The model under review builds one solid part; all positions refer to its coordinate system, in mm. Face numbers are marked on the shaded views. Coordinates: 2 decimals unless noted, no trailing zeros. Write each loop counter-clockwise with the first axis right and the second up, starting at its lowest first coordinate (ties: lowest second). Pieces come first, ordered by that corner, then holes. Notation, with made-up numbers: M 5.25,30 L 50.25,30 A10 ccw 50.25,46 Z; hole C 15.25,15.5 d6. An arc over 180 degrees is marked long. Answer as a JSON object with one key per item and string values.
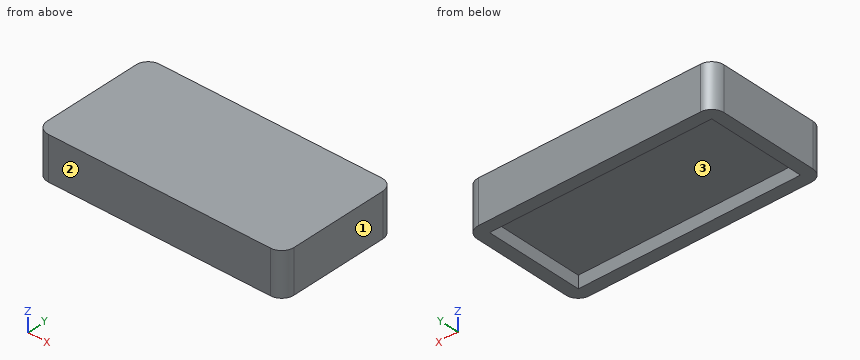
```python
from build123d import *

# Parameters (mm, degrees)
BOSS_EXTRUDE1_DEPTH = 3.5
SKETCH2_W           = 18
SKETCH2_H           = 8
CUT_EXTRUDE1_DEPTH  = 1


with BuildPart() as part:
    # Sketch1 → Boss-Extrude1 (new body)
    with BuildSketch(Plane.XY):
        with BuildLine():
            Line((-9, 5), (9, 5))
            ThreePointArc((9, 5), (9.707106781, 4.707106781), (10, 4))
            Line((10, 4), (10, -4))
            ThreePointArc((10, -4), (9.707106781, -4.707106781), (9, -5))
            Line((9, -5), (-9, -5))
            ThreePointArc((-9, -5), (-9.707106781, -4.707106781), (-10, -4))
            Line((-10, -4), (-10, 4))
            ThreePointArc((-10, 4), (-9.707106781, 4.707106781), (-9, 5))
        make_face()
    extrude(amount=BOSS_EXTRUDE1_DEPTH)

    # Sketch2 → Cut-Extrude1 (cut)
    with BuildSketch(Plane(origin=(0, 0, 0), x_dir=(-1, 0, 0), z_dir=(0, 0, -1))):
        Rectangle(SKETCH2_W, SKETCH2_H)
    extrude(amount=-CUT_EXTRUDE1_DEPTH, mode=Mode.SUBTRACT)


solid = part.part
```
(1) Add section C-C on y = 0.5. Give the boundary of the cut face in (x, z).
Results list:
{"outline": "M -10,0 L -9,0 L -9,1 L 9,1 L 9,0 L 10,0 L 10,3.5 L -10,3.5 Z"}
(2) Add section B-B on z = 0.4. Give the boundary of the cut face in (x, y), and give its area (3 significant figures).
Results list:
{"outline": "M -10,-4 A1 ccw -9,-5 L 9,-5 A1 ccw 10,-4 L 10,4 A1 ccw 9,5 L -9,5 A1 ccw -10,4 Z; hole M -9,-4 L 9,-4 L 9,4 L -9,4 Z", "area": "55.1 mm²"}
(3) Draft analysis for pull direction X (two halves, no side actions). For the marked faces 1, 2 and 3, state which applies: released by +X, released by -X, zero draft, split by the parting line, or undercut.
Results list:
{"face 1": "released by +X", "face 2": "zero draft", "face 3": "undercut"}
(4) Add section A-A on x = -4. Give the boundary of the cut face in (y, z).
Results list:
{"outline": "M -5,0 L -4,0 L -4,1 L 4,1 L 4,0 L 5,0 L 5,3.5 L -5,3.5 Z"}
(5) Wall thickness on line 1 along X through (y, z) = (-0.5, 0.5); line 2 along Y through (x, z) = (-7.25, 0.3); line 3 along Z through (x, y) = (-8.75, 1): over which ranges is each line inside the solid? List them lowest first. Write a range as from..to.
Results list:
{"line 1": "-10..-9, 9..10", "line 2": "-5..-4, 4..5", "line 3": "1..3.5"}
